```python
from build123d import *

# Parameters (mm, degrees)
F0_W     = 38.1
F0_H     = 6.35
F2_DEPTH = 8.001
F1_R     = 2.286
F3_DEPTH = 25.4
F4_R     = 2.54
F5_R     = 2.54
F6_R     = 2.54
F7_R     = 2.54


with BuildPart() as f2:
    # F0 (on Right) → F2 (new body)
    with BuildSketch(Plane.YZ):
        with Locations((1.877956, -1.010046)):
            Rectangle(F0_W, F0_H)
    extrude(amount=F2_DEPTH)

    # F1 (on face) → F3 (cut)
    with BuildSketch(Plane.YZ):
        with Locations((-13.943814, -0.854794)):
            Circle(F1_R)
        with Locations((-5.968214, -0.854794)):
            Circle(F1_R)
        with Locations((2.007386, -0.854794)):
            Circle(F1_R)
        with Locations((9.982986, -0.854794)):
            Circle(F1_R)
        with Locations((17.958586, -0.854794)):
            Circle(F1_R)
    extrude(amount=F3_DEPTH, mode=Mode.SUBTRACT)

    # F4
    f4_edges = [f2.edges().sort_by_distance(p)[0] for p in [
        (4.0005, -17.172044, 2.164954),
    ]]
    fillet(f4_edges, radius=F4_R)

    # F5
    f5_edges = [f2.edges().sort_by_distance(p)[0] for p in [
        (4.0005, -17.172044, -4.185046),
    ]]
    fillet(f5_edges, radius=F5_R)

    # F6
    f6_edges = [f2.edges().sort_by_distance(p)[0] for p in [
        (4.0005, 20.927956, 2.164954),
    ]]
    fillet(f6_edges, radius=F6_R)

    # F7
    f7_edges = [f2.edges().sort_by_distance(p)[0] for p in [
        (4.0005, 20.927956, -4.185046),
    ]]
    fillet(f7_edges, radius=F7_R)


solid = f2.part
```
For this review, take the finished solid that the model builds, in its own axes (mm). Round coordinates to 2 decimals unless told otherwise and drop trailing zeros. Loops run counter-clockwise (first coordinate to the right, second up) from the corner with the lowest first, then second, coordinate; pieces in that order, holes last.
Q1. To check wall thickness, follow line 1 along Y through (x, z) = (2, -1); line 2 along Y through (x, z) = (7.75, -0.75); line 3 along Z through (x, y) = (6.25, -5). State the ranges of each line that lie inside material, in increasing order.
Result sheet:
line 1: y = -17.17 to -16.23, -11.66 to -8.25, -3.69 to -0.27, 4.29 to 7.7, 12.26 to 15.68, 20.24 to 20.93
line 2: y = -17.17 to -16.23, -11.66 to -8.25, -3.68 to -0.28, 4.29 to 7.7, 12.27 to 15.67, 20.24 to 20.93
line 3: z = -4.19 to -2.93, 1.22 to 2.16
Q2. Add section C-C on x = 5.5. Write out the cut boundary in (y, z), plus the area to 3 significant figures.
Result sheet:
outline: (-17.17, -1.65) arc R2.54 ccw to (-14.63, -4.19) - (18.39, -4.19) arc R2.54 ccw to (20.93, -1.65) - (20.93, -0.38) arc R2.54 ccw to (18.39, 2.16) - (-14.63, 2.16) arc R2.54 ccw to (-17.17, -0.38) - close; hole circle Ø4.57 at (-13.94, -0.85); hole circle Ø4.57 at (-5.97, -0.85); hole circle Ø4.57 at (2.01, -0.85); hole circle Ø4.57 at (9.98, -0.85); hole circle Ø4.57 at (17.96, -0.85)
area: 154 mm2
Q3. Mouldability with a two-part tool opening along Y and no side actions: class faces 1 (the face through (3.94, 7.7, -0.75)), 2 (the face through (4, -17.172, -1)), 3 (the face through (8.001, 2, -4)) as +Y half, -Y half, draft (parallel to the pull), parting line (faces both ways), or undercut.
Result sheet:
face 1: undercut
face 2: -Y half
face 3: draft
Q4. Add section A-A on z = -2.5. Write out the cut boundary in (x, y), plus the area to 3 significant figures.
Result sheet:
outline: (0, -17.02) - (8, -17.02) - (8, -15.53) - (0, -15.53) - close; (0, -12.36) - (8, -12.36) - (8, -7.56) - (0, -7.56) - close; (0, -4.38) - (8, -4.38) - (8, 0.42) - (0, 0.42) - close; (0, 3.59) - (8, 3.59) - (8, 8.4) - (0, 8.4) - close; (0, 11.57) - (8, 11.57) - (8, 16.37) - (0, 16.37) - close; (0, 19.55) - (8, 19.55) - (8, 20.78) - (0, 20.78) - close
area: 175 mm2
Q5. Add section B-B on y = 9. Write out the cut boundary in (x, z), plus the area to 3 significant figures.
Result sheet:
outline: (0, -4.19) - (8, -4.19) - (8, -2.92) - (0, -2.92) - close; (0, 1.21) - (8, 1.21) - (8, 2.16) - (0, 2.16) - close
area: 17.8 mm2
Q6. Add section D-D on z = 0.75. Write out the cut boundary in (x, y).
Result sheet:
outline: (0, -16.91) - (8, -16.91) - (8, -15.57) - (0, -15.57) - close; (0, -12.32) - (8, -12.32) - (8, -7.6) - (0, -7.6) - close; (0, -4.34) - (8, -4.34) - (8, 0.38) - (0, 0.38) - close; (0, 3.64) - (8, 3.64) - (8, 8.35) - (0, 8.35) - close; (0, 11.61) - (8, 11.61) - (8, 16.33) - (0, 16.33) - close; (0, 19.59) - (8, 19.59) - (8, 20.67) - (0, 20.67) - close
